from build123d import *

# Parameters (mm, degrees)
F0_W     = 3.5
F0_H     = 3.5
F0_W_2   = 5
F0_H_2   = 12.5
F1_DEPTH = 5
F2_R     = 3


with BuildPart() as f1:
    # F0 (on Top) → F1 (new body)
    with BuildSketch(Plane.XY):
        Polygon((33.5, -32.5), (33.5, 32.5), (16, 32.5), (16, 27.5), (21, 27.5), (28.5, 27.5), (28.5, -27.5), (-28.5, -27.5), (-28.5, 27.5), (-21, 27.5), (-16, 27.5), (-16, 32.5), (-33.5, 32.5), (-33.5, -32.5), align=None)
        with Locations((-31, -27)):
            Rectangle(F0_W, F0_H, mode=Mode.SUBTRACT)
        with Locations((31, -27)):
            Rectangle(F0_W, F0_H, mode=Mode.SUBTRACT)
        with Locations((-31, 27)):
            Rectangle(F0_W, F0_H, mode=Mode.SUBTRACT)
        with Locations((31, 27)):
            Rectangle(F0_W, F0_H, mode=Mode.SUBTRACT)
        with Locations((-18.5, 21.25)):
            Rectangle(F0_W_2, F0_H_2)
        with BuildLine():
            Line((21, 15), (16, 15))
            ThreePointArc((16, 15), (0, -1), (-16, 15))
            Line((-16, 15), (-21, 15))
            ThreePointArc((-21, 15), (0, -6), (21, 15))
        make_face()
        with Locations((18.5, 21.25)):
            Rectangle(F0_W_2, F0_H_2)
    extrude(amount=F1_DEPTH)

    # F2
    f2_edges = [f1.edges().sort_by_distance(p)[0] for p in [
        (-33.5, 32.5, 2.5),
        (-16, 32.5, 2.5),
        (16, 32.5, 2.5),
        (33.5, 32.5, 2.5),
        (-28.5, 27.5, 2.5),
        (-21, 27.5, 2.5),
        (21, 27.5, 2.5),
        (28.5, 27.5, 2.5),
        (28.5, -27.5, 2.5),
        (-28.5, -27.5, 2.5),
        (33.5, -32.5, 2.5),
        (-33.5, -32.5, 2.5),
    ]]
    fillet(f2_edges, radius=F2_R)


solid = f1.part
The listing builds one solid part. Answer for the finished solid, in the listing's coordinates (mm). A direction names the side the tool comes from. Give positions to 0.01 mm unless a question says otherwise; leave off trailing zeros. Order: outer loops, then holes, each group sorted by start corner. A loop starts at its lowest first (then second) coordinate and runs counter-clockwise, first axis right, second up. Notation, with made-up numbers: (-34, -19) -> (6, -19) arc R22 cw to (6, -8) -> close; hole circle Ø2 at (-31, -29). An arc over 180 degrees is marked (long way). Put each result on its own line as item: value.
Item 1: A cutting plane is placed at C-C on z = 2.6. Count the separate pieces of the cut face and the enclosed holes in it, plus the area to 3 significant figures.
Established:
separate pieces: 1
enclosed holes: 5
area: 1,430 mm^2
Item 2: Given P1, Ø1.5, axis at x = 4.5, z = 2, coming from the +Y side; P2, Ø1, axis at x = -3.5, z = 3.5, coming from the +Y side; P3, Ø1, axis at x = -5.5, z = 1, coming from the +Y side, each flat-ended and moving along its own axis, determine where each tip first touches the part or whether it passes through.
Established:
P1: stops at y = -0.11
P2: stops at y = -0.49
P3: stops at y = 0.17
Item 3: A cutting plane is placed at A-A on y = -16. Give the vertices of the cut face in (x, z).
Established:
outline: (-33.5, 0) -> (-28.5, 0) -> (-28.5, 5) -> (-33.5, 5) -> close; (28.5, 0) -> (33.5, 0) -> (33.5, 5) -> (28.5, 5) -> close
Item 4: Straight lines are drawn through the part: line 1 (X direction, y = 18.5, z = 4.6); line 2 (X direction, y = 10.5, z = 3.6); line 3 (Y direction, x = 30, z = 2.3). For each, find the intervals that lie inside material, in ascending order.
Established:
line 1: x = -33.5 to -28.5, -21 to -16, 16 to 21, 28.5 to 33.5
line 2: x = -33.5 to -28.5, -20.51 to -15.35, 15.35 to 20.51, 28.5 to 33.5
line 3: y = -32.5 to -28.75, -25.25 to 25.25, 28.75 to 32.5
Item 5: For faces 4 (the face through (29.25, 27, 2)), 5 (the face through (16.9, 31.64, 2.54)), 6 (the face through (-33.5, 0, 2)), determine the directions among +Z, -Z, +X, -X, +Y, -Y from which every point of the face is accessible in a straight line to the end or side of a thin tool.
Established:
face 4: +Z, -Z
face 5: +Z, -Z, +Y
face 6: +Z, -Z, -X, +Y, -Y
Item 6: A cutting plane is placed at B-B on x = 0. Give the vertices of the cut face in (y, z), plus the area to 3 significant figures.
Established:
outline: (-32.5, 0) -> (-27.5, 0) -> (-27.5, 5) -> (-32.5, 5) -> close; (-6, 0) -> (-1, 0) -> (-1, 5) -> (-6, 5) -> close
area: 50.0 mm^2
Item 7: For a pull along Y with two mould halves and no side action, classify faces 1 (the face through (-31, -25.25, 2)), 2 (the face through (25, 32.5, 2)), 3 (the face through (-32.64, -31.6, 2.54)) as released by +Y, released by -Y, zero draft, split by the parting line, or undercut.
Established:
face 1: undercut
face 2: released by +Y
face 3: released by -Y
